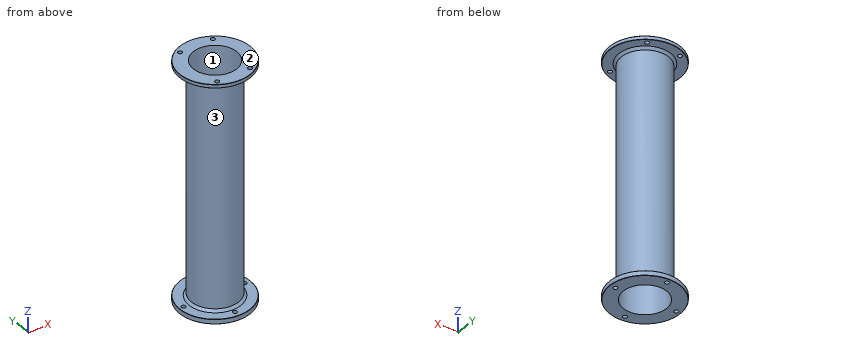
```python
from build123d import *

# Parameters (mm, degrees)
SKIZZE1_R                       = 150
SKIZZE1_R_2                     = 92
SKIZZE1_R_3                     = 9
AUFSATZ_LINEAR_AUSTRAGEN1_DEPTH = 20
SKIZZE2_R                       = 100
SKIZZE2_R_2                     = 92
AUFSATZ_LINEAR_AUSTRAGEN2_DEPTH = 965
SKIZZE3_R                       = 150
SKIZZE3_R_2                     = 92
SKIZZE3_R_3                     = 9
AUFSATZ_LINEAR_AUSTRAGEN3_DEPTH = 15
FASE1_SIZE                      = 10
FASE2_SIZE                      = 1


with BuildPart() as part:
    # Skizze1 → Aufsatz-Linear austragen1 (new body)
    with BuildSketch(Plane.XY):
        Circle(SKIZZE1_R)
        Circle(SKIZZE1_R_2, mode=Mode.SUBTRACT)
        with Locations((0, 130)):
            Circle(SKIZZE1_R_3, mode=Mode.SUBTRACT)
        with Locations((125, 0)):
            Circle(SKIZZE1_R_3, mode=Mode.SUBTRACT)
        with Locations((-5, -125)):
            Circle(SKIZZE1_R_3, mode=Mode.SUBTRACT)
        with Locations((-130, 5)):
            Circle(SKIZZE1_R_3, mode=Mode.SUBTRACT)
    extrude(amount=AUFSATZ_LINEAR_AUSTRAGEN1_DEPTH)

    # Skizze2 → Aufsatz-Linear austragen2 (add)
    with BuildSketch(Plane.XY.offset(20)):
        Circle(SKIZZE2_R)
        Circle(SKIZZE2_R_2, mode=Mode.SUBTRACT)
    extrude(amount=AUFSATZ_LINEAR_AUSTRAGEN2_DEPTH)

    # Skizze3 → Aufsatz-Linear austragen3 (add)
    with BuildSketch(Plane.XY.offset(985)):
        Circle(SKIZZE3_R)
        Circle(SKIZZE3_R_2, mode=Mode.SUBTRACT)
        with Locations((-70, 110)):
            Circle(SKIZZE3_R_3, mode=Mode.SUBTRACT)
        with Locations((70, 110)):
            Circle(SKIZZE3_R_3, mode=Mode.SUBTRACT)
        with Locations((70, -110)):
            Circle(SKIZZE3_R_3, mode=Mode.SUBTRACT)
        with Locations((-70, -110)):
            Circle(SKIZZE3_R_3, mode=Mode.SUBTRACT)
    extrude(amount=AUFSATZ_LINEAR_AUSTRAGEN3_DEPTH)

    # Fase1
    fase1_edges = [part.edges().sort_by_distance(p)[0] for p in [
        (-100, 0, 985),
        (-100, 0, 20),
    ]]
    chamfer(fase1_edges, length=FASE1_SIZE)

    # Fase2
    fase2_edges = [part.edges().sort_by_distance(p)[0] for p in [
        (-150, 0, 0),
        (-150, 0, 1000),
        (-150, 0, 985),
        (-150, 0, 20),
    ]]
    chamfer(fase2_edges, length=FASE2_SIZE)


solid = part.part
```
Input: part model. Units: mm. Frame: model coordinates. Face numbers are marked on the shaded views. Round coordinates to 2 decimals unless told otherwise and drop trailing zeros. Order: outer loops, then holes, each group sorted by start corner. A loop starts at its lowest first (then second) coordinate and runs counter-clockwise, first axis right, second up. Notation, with made-up numbers: (-6, 13.25) - (18, 13.25) arc R15 cw to (18, 35.25) - close; hole circle Ø2 at (54, -8). An arc over 180 degrees is marked (long way). Answer in a Markdown table with one row per item.
Item 1: Line query: line 1 (Y direction, x = -1.5, z = 349); line 2 (Z direction, x = 112.5, y = 75); line 3 (Y direction, x = 70, z = 995) (3 decimals). Output: solid intervals per line, ascending.
Model answer:
| item | result |
|---|---|
| line 1 | y = -99.99 to -91.99, 91.99 to 99.99 |
| line 2 | z = 0 to 20, 985 to 1000 |
| line 3 | y = -132.665 to -119, -101 to -59.699, 59.699 to 101, 119 to 132.665 |
Item 2: Section query A-A (z = 155). Return the cut outline in (x, y), then the cut area to 3 significant figures.
Model answer:
| item | result |
|---|---|
| outline | circle Ø200 at (0, 0); hole circle Ø184 at (0, 0) |
| area | 4,830 mm² |
Item 3: Pin query (flat end, axial travel): pin 1 (4 mm diameter, centred on x = 5, z = 266.5, fed in from +Y) (3 decimals); pin 2 (1.5 mm diameter, centred on x = -87.5, z = 610, fed in from -Y); pin 3 (16 mm diameter, centred on x = 0, y = 130, fed in from -Z); pin 4 (16 mm diameter, centred on x = 70, y = -110, fed in from -Z). Return the tip coordinate at first contact, or that it passes through.
Model answer:
| item | result |
|---|---|
| pin 1 | stops at y = 99.955 |
| pin 2 | stops at y = -49.74 |
| pin 3 | stops at z = 985 |
| pin 4 | stops at z = 0 |
Item 4: Mould query, pull axis X, two halves, no side actions, for the marked faces 1, 2 and 3. Classes: released by +X, released by -X, zero draft, split by the parting line, or undercut.
Model answer:
| item | result |
|---|---|
| face 1 | undercut |
| face 2 | zero draft |
| face 3 | split by the parting line |
Item 5: Section query B-B (y = 130). Give the number of separate pieces and of enclosed holes in the cut face, then the cut area to 3 significant figures.
Model answer:
| item | result |
|---|---|
| separate pieces | 3 |
| enclosed holes | 0 |
| area | 4,870 mm² |
